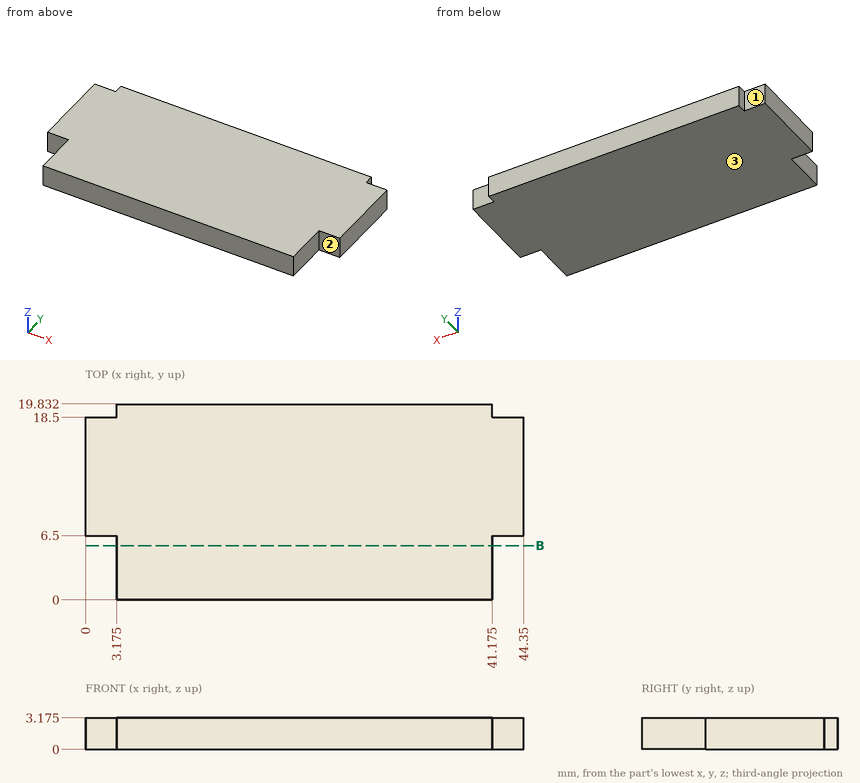
Design review of the part shown in the three views and the two pictorial views. Dimensions are in mm from the part's minimum x, y and z. A direction names the side the tool comes from. Give positions to 0.01 mm unless a question says otherwise; leave off trailing zeros. Write each loop counter-clockwise with the first axis right and the second up, starting at its lowest first coordinate (ties: lowest second). Pieces come first, ordered by that corner, then holes. Notation, with made-up numbers: M 15,-22 L 39,-22 A19 cw 39,12 Z; hole C 25.5,-9.5 d11. An arc over 180 degrees is marked long. One line per item, written item: value.
1) For line 1 (X direction, y = 5, z = 2.55) (1 decimal), list the stretches that pass through material, from the lowest coordinate up. Write a range as from..to.
Results are:
line 1: x = 3.2..41.2
2) For the marked faces 1, 2 and 3, list the 3-axis set-ups (+Z, -Z, +X, -X, +Y, -Y) from which the entire face can be reached by the end or side of a thin tool; tool diameter is ignored.
Results are:
face 1: +Z, -Z, -X, +Y
face 2: +Z, -Z, +X, -Y
face 3: -Z, +X, -X, +Y, -Y
3) For P1, Ø1.6, axis at x = 1.5, z = 2, coming from the +Y side; P2, Ø1, axis at y = 4.5, z = 1.5, coming from the +X side (3 decimals); P3, Ø1, axis at x = 43.5, z = 2.5, coming from the -Y side, all flat-tipped, find the tip position at first contact; note any pin that passes through.
Results are:
P1: stops at y = 18.5
P2: stops at x = 41.175
P3: stops at y = 6.5
4) Take a section at B-B, the plane y = 5.5. Write out the cut boundary in (x, z) (1 decimal).
Results are:
outline: M 3.2,0 L 41.2,0 L 41.2,3.2 L 3.2,3.2 Z
